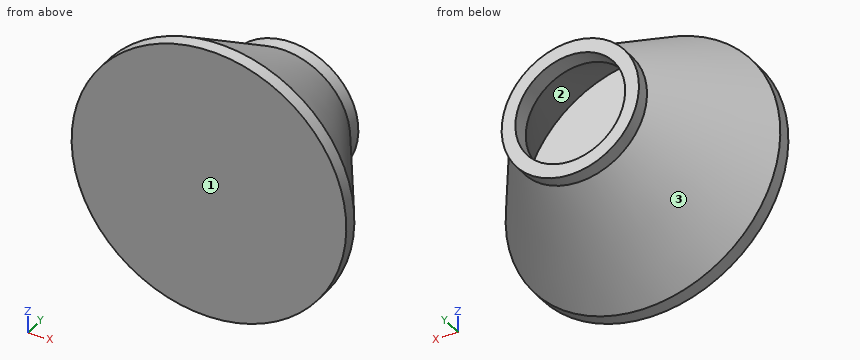
from build123d import *

# Parameters (mm, degrees)
SHELL1_T = -10


with BuildPart() as part:
    # Sketch2 → Revolve1 (revolve)
    with BuildSketch(Plane.XY, mode=Mode.PRIVATE) as revolve1_sk:
        Polygon((0, 0), (100, 0), (100, 10), (50, 90), (50, 100), (0, 100), align=None)
    revolve(revolve1_sk.sketch.rotate(Axis((0, 0, 0), (0, 1, 0)), 90), axis=Axis((0, 0, 0), (0, 1, 0)))

    # Shell1
    shell1_openings = [part.faces().sort_by_distance(p)[0] for p in [
        (0, 100, 0),
    ]]
    offset(amount=SHELL1_T, openings=shell1_openings, kind=Kind.INTERSECTION)


solid = part.part
Model file for the job. Use its own axes, mm. Face numbers are marked on the shaded views. Coordinates: 2 decimals unless noted, no trailing zeros. Order: outer loops, then holes, each group sorted by start corner. A loop starts at its lowest first (then second) coordinate and runs counter-clockwise, first axis right, second up. Notation, with made-up numbers: M 60,26.25 L 76,26.25 A36 cw 76,63.25 Z; hole C 24,31 d2. An arc over 180 degrees is marked long. Return JSON: item names as keys, results as strings.
1. Saw through at D-D (y = 7). Give the cut face in (x, z).
Ans:
{"outline": "C 0,0 d200"}
2. Saw through at A-A (x = 0). Give the cut face in (y, z).
Ans:
{"outline": "M 0,-100 L 10,-100 L 90,-50 L 100,-50 L 100,-40 L 87.13,-40 L 10,-88.21 L 10,88.21 L 87.13,40 L 100,40 L 100,50 L 90,50 L 10,100 L 0,100 Z"}
3. Saw through at C-C (y = 50). Give the cut face in (x, z), and give its area (3 significant figures).
Ans:
{"outline": "C 0,0 d150; hole C 0,0 d126.42", "area": "5,120 mm^2"}
4. Flat gauge pins, fed straight in: pin 1 (1 mm diameter, centred on y = 68.5, z = -34, fed in from +X); pin 2 (1 mm diameter, centred on y = 15, z = -65, fed in from -X); pin 3 (8 mm diameter, centred on x = -30, z = 5.5, fed in from +Y); pin 4 (4 mm diameter, centred on x = -23.5, z = 19.5, fed in from -Y). Where does each tip first touch, or does it go through?
Ans:
{"pin 1": "x = 54.04", "pin 2": "x = -72.45", "pin 3": "y = 10", "pin 4": "y = 0"}
5. Drill centre lines: probe 1 along X at (y, z) = (90, 0); probe 2 along Z at (x, y) = (-42.5, 12); probe 3 along Y at (x, z) = (56.5, -31). Where is each one in solid material? Low to high.
Ans:
{"probe 1": "-50 to -40, 40 to 50", "probe 2": "-89.14 to -75.86, 75.86 to 89.14", "probe 3": "0 to 10, 48.02 to 66.89"}
6. Pull direction X, two halves, no side cores. Call the marked faces 1, 2 and 3: +X half, -X half, draft (parallel to the pull), parting line (faces both ways), or undercut.
Ans:
{"face 1": "draft", "face 2": "undercut", "face 3": "parting line"}
7. Saw through at B-B (z = 0). Give the cut face in (x, y), and give its area (3 significant figures).
Ans:
{"outline": "M -100,0 L 100,0 L 100,10 L 50,90 L 50,100 L 40,100 L 40,87.13 L 88.21,10 L -88.21,10 L -40,87.13 L -40,100 L -50,100 L -50,90 L -100,10 Z", "area": "4,080 mm^2"}
